```python
from build123d import *
from build123d.topology import SkipClean

# Parameters (mm, degrees)
SZKIC1_R                    = 4
DODANIE_WYCI_GNI_CIE1_DEPTH = 110
ZAOKR_GLENIE6_R             = 4
WYTNIJ_WYCI_GNI_CIE4_START  = -2
SZKIC2_W                    = 8
SZKIC2_H                    = 10
WYTNIJ_WYCI_GNI_CIE4_DEPTH  = 2
WYTNIJ_WYCI_GNI_CIE5_START  = -4
SZKIC5_W                    = 6.92820323
SZKIC5_H                    = 10
WYTNIJ_WYCI_GNI_CIE5_DEPTH  = 2
WYTNIJ_WYCI_GNI_CIE6_REACH  = 112.236
SZKIC6_R                    = 2
DODANIE_WYCI_GNI_CIE2_START = 7
SZKIC8_R                    = 4
DODANIE_WYCI_GNI_CIE2_DEPTH = 7
ZAOKR_GLENIE7_R             = 4


with BuildPart() as part:
    # Szkic1 → Dodanie-wyci_gni_cie1 (new body)
    with BuildSketch(Plane.XY):
        Circle(SZKIC1_R)
    extrude(amount=DODANIE_WYCI_GNI_CIE1_DEPTH)

    # Zaokr_glenie6
    zaokr_glenie6_edges = [part.edges().sort_by_distance(p)[0] for p in [
        (-4, 0, 110),
    ]]
    fillet(zaokr_glenie6_edges, radius=ZAOKR_GLENIE6_R)

    # Szkic2 → Wytnij-wyci_gni_cie4 (cut)
    with BuildSketch(Plane(origin=(0, 0, 0), x_dir=(1, 0, 0), z_dir=(0, 1, 0)).offset(WYTNIJ_WYCI_GNI_CIE4_START)):
        with Locations((0, -105)):
            Rectangle(SZKIC2_W, SZKIC2_H)
    extrude(amount=-WYTNIJ_WYCI_GNI_CIE4_DEPTH, mode=Mode.SUBTRACT)

    # Szkic5 → Wytnij-wyci_gni_cie5 (cut)
    with BuildSketch(Plane.XZ.offset(2).offset(WYTNIJ_WYCI_GNI_CIE5_START)):
        with Locations((0, 105)):
            Rectangle(SZKIC5_W, SZKIC5_H)
    extrude(amount=-WYTNIJ_WYCI_GNI_CIE5_DEPTH, mode=Mode.SUBTRACT)

    # Szkic6 → Wytnij-wyci_gni_cie6 (cut, up to next)
    with BuildSketch(Plane.XZ.offset(2), mode=Mode.PRIVATE) as wytnij_wyci_gni_cie6_sk1:
        with Locations(Location((0, 105, 0), (0, 0, 270))):
            Circle(SZKIC6_R)
    wytnij_wyci_gni_cie6_tool1 = extrude(wytnij_wyci_gni_cie6_sk1.sketch, amount=-WYTNIJ_WYCI_GNI_CIE6_REACH, mode=Mode.PRIVATE) & part.part
    add(wytnij_wyci_gni_cie6_tool1.solids().sort_by_distance((0, -2, 105))[0], mode=Mode.SUBTRACT)

    # Szkic8 → Dodanie-wyci_gni_cie2 (add)
    with SkipClean():  # the faces are left unmerged after this step: merging them gives an invalid solid
        with BuildSketch(Plane(origin=(0, 0, 0), x_dir=(-1, 0, 0), z_dir=(0, 0, -1)).offset(DODANIE_WYCI_GNI_CIE2_START)):
            Circle(SZKIC8_R)
        extrude(amount=-DODANIE_WYCI_GNI_CIE2_DEPTH)

    # Zaokr_glenie7
    zaokr_glenie7_edges = [part.edges().sort_by_distance(p)[0] for p in [
        (4, 0, -7),
    ]]
    fillet(zaokr_glenie7_edges, radius=ZAOKR_GLENIE7_R)


solid = part.part
```
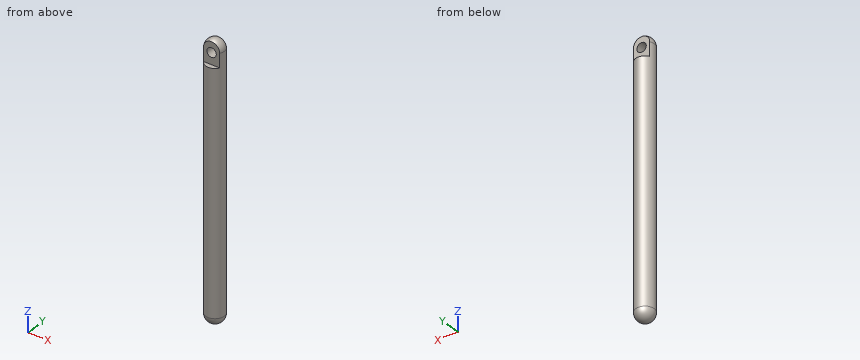
Geometry check sheet. Reference: the model listing, model coordinates, mm. Coordinates: 2 decimals unless noted, no trailing zeros. Write each loop counter-clockwise with the first axis right and the second up, starting at its lowest first coordinate (ties: lowest second). Pieces come first, ordered by that corner, then holes. Notation, with made-up numbers: M -18,54 L 37,54 A25 ccw 37,66 Z; hole C 12,73.25 d9. An arc over 180 degrees is marked long. Answer as a JSON object with one key per item and string values.
1. Section check D-D, the plane z = 7. Enter the section's corners in (x, y), plus the area to 3 significant figures.
Answers below:
{"outline": "C 0,0 d8", "area": "50.3 mm²"}
2. Scan lines: L1, parallel to Z at x = 0.25, y = -0.25; L2, parallel to X at y = 0.2, z = 105 (3 decimals); L3, parallel to X at y = 0.25, z = 71.5. Record each from-to range of solid material in increasing order.
Answers below:
{"L1": "z = -6.98 to 103.02, 106.98 to 109.98", "L2": "x = -3.995 to -2, 2 to 3.995", "L3": "x = -3.99 to 3.99"}
3. Section check C-C, the plane y = 1. Enter the section's corners in (x, z).
Answers below:
{"outline": "M -3.87,-3 A3.87 ccw 3.87,-3 L 3.87,106 A3.87 ccw -3.87,106 Z; hole C 0,105 d4"}
4. Section check A-A, the plane x = 0. Enter the section's corners in (y, z).
Answers below:
{"outline": "M -4,-3 A4 ccw 4,-3 L 4,100 L 2,100 L 2,103 L -2,103 L -2,100 L -4,100 Z; M -2,107 L 2,107 L 2,109.46 A4 ccw -2,109.46 Z"}
5. Go/stop test with flat-tipped pins: pin 1 Ø2 at (y, z) = (-1.5, 66) entering from +X; pin 2 Ø1.5 at (x, z) = (3, 81) entering from +Y; pin 3 Ø2 at (x, y) = (0, 2.5) entering from +Z; pin 4 Ø2.5 at (x, z) = (0, 105) entering from -Y. Record where each tip stops, or that it passes through.
Answers below:
{"pin 1": "stops at x = 3.97", "pin 2": "stops at y = 3.31", "pin 3": "stops at z = 109.71", "pin 4": "passes through"}
6. Section check B-B, the plane z = 105. Enter the section's corners in (x, y), plus the area to 3 significant figures.
Answers below:
{"outline": "M -3.46,-2 L -2,-2 L -2,2 L -3.46,2 A4 ccw Z; M 2,-2 L 3.46,-2 A4 ccw 3.46,2 L 2,2 Z", "area": "14.6 mm²"}
